The model under review builds one solid part; all positions refer to its coordinate system, in mm. Face numbers are marked on the shaded views. A direction names the side the tool comes from. Give positions to 0.01 mm unless a question says otherwise; leave off trailing zeros. Order: outer loops, then holes, each group sorted by start corner. A loop starts at its lowest first (then second) coordinate and runs counter-clockwise, first axis right, second up. Notation, with made-up numbers: (69.25, 64) - (76.25, 64) arc R16 cw to (76.25, 89) - close; hole circle Ø5 at (6, 86). An arc over 180 degrees is marked (long way). Use CSV: the item, a comma, the result in double quotes. Start each with the question number.
1. Take a section at C-C, the plane y = 198. State the section outline as (x, z) points.
2. Take a section at B-B, the plane x = 8.75. State the section outline as (y, z) points.
3. Draft analysis for pull direction Z (two halves, no side actions). For the marked faces 3, 4 and 5, state which applies: released by +Z, released by -Z, zero draft, split by the parting line, or undercut.
4. To check wall thickness, follow line 1 (Y direction, x = 14.25, z = 0); line 2 (Z direction, x = 11, y = 88). State the ranges of each line that lie inside material, in increasing order. Write a range as [from, to].
5. Take a section at A-A, the plane z = -5.25. State the section outline as (x, y) points.
6. For pin 1 (1 mm diameter, centred on x = 11.5, z = 11.5, fed in from -Y), flat-tipped, find the tip position at first contact; note if it passes through.
7. Machinability: for the marked faces 1 and 2, which of the approach directions +Z, -Z, +X, -X, +Y, -Y give a long, thin tool a straight path to every point of the face, cutting with its end or side? Answer none if there is none.
```python
from build123d import *

# Parameters (mm, degrees)
BOSS_EXTRUDE1_DEPTH = 245
SKETCH2_W           = 26
SKETCH2_H           = 26
CUT_EXTRUDE1_DEPTH  = 245
SKETCH4_R           = 3
CUT_EXTRUDE3_DEPTH  = 30


with BuildPart() as part:
    # Sketch1 → Boss-Extrude1 (new body)
    with BuildSketch(Plane(origin=(0, 0, 0), x_dir=(1, 0, 0), z_dir=(0, 1, 0))):
        Polygon((-15, 0), (-15, 15), (15, 15), (15, -15), (-15, -15), align=None)
    extrude(amount=BOSS_EXTRUDE1_DEPTH)

    # Sketch2 → Cut-Extrude1 (cut)
    with BuildSketch(Plane(origin=(0, 245, 0), x_dir=(1, 0, 0), z_dir=(0, 1, 0))):
        Rectangle(SKETCH2_W, SKETCH2_H)
    extrude(amount=-CUT_EXTRUDE1_DEPTH, mode=Mode.SUBTRACT)

    # Sketch4 → Cut-Extrude3 (cut)
    with BuildSketch(Plane.ZY.offset(15)):
        with Locations((0, 205)):
            Circle(SKETCH4_R)
        with Locations((0, 185)):
            Circle(SKETCH4_R)
        with Locations((0, 60)):
            Circle(SKETCH4_R)
        with Locations((0, 40)):
            Circle(SKETCH4_R)
    extrude(amount=-CUT_EXTRUDE3_DEPTH, mode=Mode.SUBTRACT)


solid = part.part
```
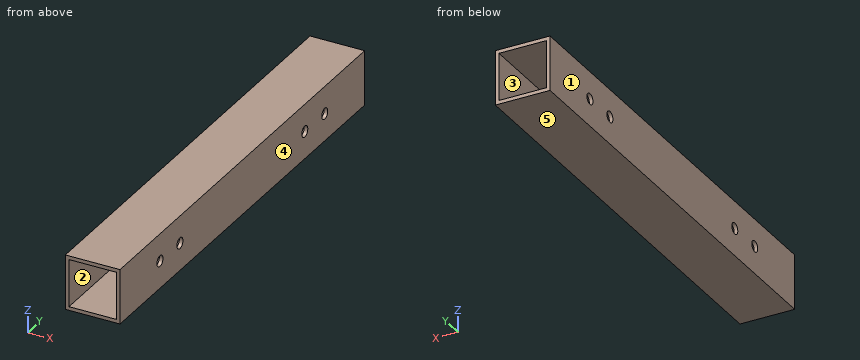
Determined:
1,outline,"(-15, -15) - (15, -15) - (15, 15) - (-15, 15) - close; hole (-13, -13) - (13, -13) - (13, 13) - (-13, 13) - close"
2,outline,"(0, -15) - (245, -15) - (245, -13) - (0, -13) - close; (0, 13) - (245, 13) - (245, 15) - (0, 15) - close"
3,face 3,"undercut"
3,face 4,"zero draft"
3,face 5,"released by -Z"
4,line 1,"y = [0, 37], [43, 57], [63, 182], [188, 202], [208, 245]"
4,line 2,"z = [-15, -13], [13, 15]"
5,outline,"(-15, 0) - (-13, 0) - (-13, 245) - (-15, 245) - close; (13, 0) - (15, 0) - (15, 245) - (13, 245) - close"
6,pin 1,"passes through"
7,face 1,"+Z, -Z, -X, +Y, -Y"
7,face 2,"+Y, -Y"
